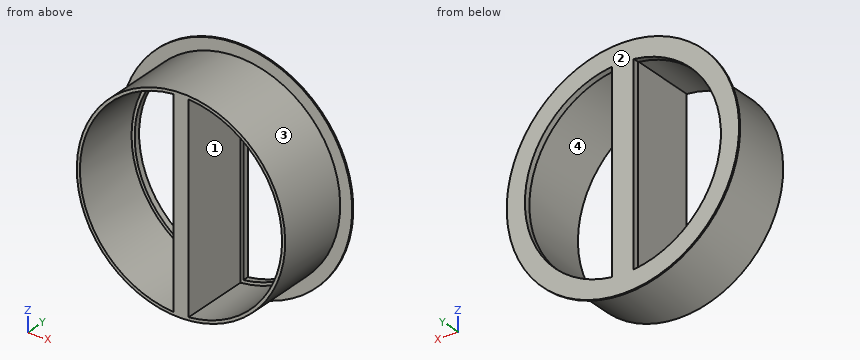
from build123d import *

# Parameters (mm, degrees)
OUTER_BASE_CIRCLE_SKETCH_R         = 37.585
BODY_EXTRUDE_DEPTH                 = 25
INNER_BASE_CIRCLE_SKETCH_OUTSIDE_W = 99.012
INNER_BASE_CIRCLE_SKETCH_OUTSIDE_H = 99.012
INNER_BASE_CIRCLE_SKETCH_OUTSIDE_R = 33.7
OUTER_BODY_EXTRUDE_DEPTH           = 24.5
DELIVERY_HOLE_EXTRUDE_DEPTH        = 59.738951727
FASTENER_EXTRUDE_DEPTH             = 23


with BuildPart() as part:
    # Outer Base Circle Sketch → Body Extrude (new body)
    with BuildSketch(Plane(origin=(0, 0, 0), x_dir=(1, 0, 0), z_dir=(0, 1, 0))):
        with Locations(Location((0, 0, 0), (0, 0, 270))):
            Circle(OUTER_BASE_CIRCLE_SKETCH_R)
    extrude(amount=BODY_EXTRUDE_DEPTH)

    # Inner Base Circle Sketch outside → Outer Body Extrude (cut)
    with BuildSketch(Plane.XZ):
        Rectangle(INNER_BASE_CIRCLE_SKETCH_OUTSIDE_W, INNER_BASE_CIRCLE_SKETCH_OUTSIDE_H)
        with Locations(Location((0, 0, 0), (0, 0, 270))):
            Circle(INNER_BASE_CIRCLE_SKETCH_OUTSIDE_R, mode=Mode.SUBTRACT)
    extrude(amount=-OUTER_BODY_EXTRUDE_DEPTH, mode=Mode.SUBTRACT)

    # Delivery Hole Sketch → Delivery Hole Extrude (cut, through all)
    with BuildSketch(Plane(origin=(0, 25, 0), x_dir=(1, 0, 0), z_dir=(0, 1, 0))):
        with BuildLine():
            Line((-3.5, 31.506189868), (-3.5, -31.506189868))
            ThreePointArc((-3.5, -31.506189868), (-31.7, 0), (-3.5, 31.506189868))
        make_face()
        with BuildLine():
            Line((3.5, 31.506189868), (3.5, -31.506189868))
            ThreePointArc((3.5, -31.506189868), (31.7, 0), (3.5, 31.506189868))
        make_face()
    extrude(amount=-DELIVERY_HOLE_EXTRUDE_DEPTH, mode=Mode.SUBTRACT)

    # Fastener Sketch → Fastener Extrude (cut)
    with BuildSketch(Plane.XZ):
        with BuildLine():
            Line((-2.5, 32.604294196), (-2.5, -32.604294196))
            ThreePointArc((-2.5, -32.604294196), (-32.7, 0), (-2.5, 32.604294196))
        make_face()
        with BuildLine():
            Line((2.5, 32.604294196), (2.5, -32.604294196))
            ThreePointArc((2.5, -32.604294196), (32.7, 0), (2.5, 32.604294196))
        make_face()
    extrude(amount=-FASTENER_EXTRUDE_DEPTH, mode=Mode.SUBTRACT)


solid = part.part
Verification items for the finished model (mm, model axes). Face numbers are marked on the shaded views. Coordinates: 2 decimals unless noted, no trailing zeros. Loops run counter-clockwise (first coordinate to the right, second up) from the corner with the lowest first, then second, coordinate; pieces in that order, holes last. Notation, with made-up numbers: (49.5, 49.5) -> (83.5, 49.5) arc R29 cw to (83.5, 79.5) -> close; hole circle Ø6 at (40.5, 34). An arc over 180 degrees is marked (long way). Write each question's results on one line, items separated by ' | '.
Item 1: Material ranges on L1, parallel to X at y = 7, z = -1; L2, parallel to X at y = 1.5, z = -26; L3, parallel to Z at x = -11, y = 6.25, recorded low to high.
Found:
L1: x = -33.69 to -32.68, -2.5 to 2.5, 32.68 to 33.69 | L2: x = -21.44 to -19.83, -2.5 to 2.5, 19.83 to 21.44 | L3: z = -31.85 to -30.79, 30.79 to 31.85
Item 2: Section check A-A, the plane z = 0. Enter the section's corners in (x, y) (3 decimals), plus the area to 3 significant figures.
Found:
outline: (-37.585, 24.5) -> (-33.7, 24.5) -> (-33.7, 0) -> (-32.7, 0) -> (-32.7, 23) -> (-31.7, 23) -> (-31.7, 25) -> (-37.585, 25) -> close; (-3.5, 23) -> (-2.5, 23) -> (-2.5, 0) -> (2.5, 0) -> (2.5, 23) -> (3.5, 23) -> (3.5, 25) -> (-3.5, 25) -> close; (31.7, 23) -> (32.7, 23) -> (32.7, 0) -> (33.7, 0) -> (33.7, 24.5) -> (37.585, 24.5) -> (37.585, 25) -> (31.7, 25) -> close | area: 187 mm2
Item 3: Mould release check, pull along X, two halves, no side actions. Record for the marked faces 1, 2, 3 and 4: +X half, -X half, draft (parallel to the pull), parting line (faces both ways), or undercut.
Found:
face 1: undercut | face 2: draft | face 3: parting line | face 4: undercut
Item 4: Gauge pin test, flat ends, axial feed: pin 1 (5 mm diameter, centred on y = 3.5, z = -12, fed in from -X); pin 2 (1.6 mm diameter, centred on y = 24.5, z = -5.5, fed in from -X); pin 3 (8 mm diameter, centred on y = 12.5, z = -8, fed in from -X). Record the tip position at first contact, or that the pin passes through.
Found:
pin 1: stops at x = -32.33 | pin 2: stops at x = -37.29 | pin 3: stops at x = -33.46
Item 5: Section check C-C, the plane x = 0. Enter the section's corners in (y, z) (3 decimals).
Found:
outline: (0, -33.7) -> (24.5, -33.7) -> (24.5, -37.585) -> (25, -37.585) -> (25, 37.585) -> (24.5, 37.585) -> (24.5, 33.7) -> (0, 33.7) -> close
Item 6: Section check B-B, the plane x = -15. Enter the section's corners in (y, z).
Found:
outline: (0, -30.18) -> (24.5, -30.18) -> (24.5, -34.46) -> (25, -34.46) -> (25, -27.93) -> (23, -27.93) -> (23, -29.06) -> (0, -29.06) -> close; (0, 29.06) -> (23, 29.06) -> (23, 27.93) -> (25, 27.93) -> (25, 34.46) -> (24.5, 34.46) -> (24.5, 30.18) -> (0, 30.18) -> close
